Can you work these out from the model? Positions are in its coordinate system, mm. A direction names the side the tool comes from. Coordinates: 2 decimals unless noted, no trailing zeros. Order: outer loops, then holes, each group sorted by start corner. A loop starts at its lowest first (then second) coordinate and runs counter-clockwise, first axis right, second up. Notation, with made-up numbers: (51, -27.75) -> (109, -27.75) arc R27 ccw to (109, -9.75) -> close; hole circle Ø10 at (-32, 13.5). An arc over 180 degrees is marked (long way). Use a Markdown table: item, result. Add a question column.
1. For faces 1 (the conical face through (-34.713, -10.932, 38.782)), 2 (the flat face through (0, 0, 1.5)), 3 (the conical face through (-20.062, 38.572, 136.423)), which set-ups out of +Z, -Z, +X, -X, +Y, -Y let a thin tool reach every point of the face, with its end or its side?
2. Suppose I cut it at A-A, the plane z = 139. List the corners of the cut face in (x, y) for me.
3. We'd pull the mould along X, two halves only. Please class faces 4 (the conical face through (-38.15, 15.82, 81.86)), 5 (the flat face through (-21, -33, 160)), 6 (the conical face through (-38.22, -12.04, 82.72)): pulls with the +X half, pulls with the -X half, needs draft (parallel to the pull), parting line crosses it, or undercut.
4. For pin 1 Ø19 at (x, y) = (-11, -14.5) entering from +Z; pin 2 Ø12 at (y, z) = (-14.5, 39.5) entering from +X; pin 3 Ø1 at (y, z) = (9.5, 140) entering from +X, each with a flat end and sliding along its axis, tell me the tip position at first contact or that it passes through.
5. If I drill on line 1 along Z through (x, y) = (23, 8); line 2 along Y through (x, z) = (-31.5, 91); line 3 along X through (y, z) = (31.5, 58.5), over which ranges is the centre line in solid material (lowest first)? Write a range as from..to.
6. Suppose I cut it at B-B, the plane z = 31. List the corners of the cut face in (x, y) for me, then the cut area to 3 significant figures.
```python
from build123d import *

# Parameters (mm, degrees)
F2_R = 5
F3_T = -1.5


with BuildPart() as f1:
    # F0 (on Front) → F1 (revolve)
    with BuildSketch(Plane.XZ):
        Polygon((-40, 80), (-33.0009069179, 0), (0, 0), (0, 160), (-40, 160), (-53.0446591225, 98.6297039244), align=None)
    revolve(axis=Axis((0, 0, 80), (0, 0, 1)))

    # F2
    f2_edges = [f1.edges().sort_by_distance(p)[0] for p in [
        (53.044659, 0, 98.629704),
        (40, 0, 80),
    ]]
    fillet(f2_edges, radius=F2_R)

    # F3
    f3_openings = [f1.faces().sort_by_distance(p)[0] for p in [
        (0, 0, 160),
    ]]
    offset(amount=F3_T, openings=f3_openings)


solid = f1.part
```
Worked out:
| question | item | result |
|---|---|---|
| 1 | face 1 | -Z |
| 1 | face 2 | +Z |
| 1 | face 3 | none |
| 2 | outline | circle Ø88.93 at (0, 0); hole circle Ø85.86 at (0, 0) |
| 3 | face 4 | parting line crosses it |
| 3 | face 5 | needs draft |
| 3 | face 6 | undercut |
| 4 | pin 1 | stops at z = 1.5 |
| 4 | pin 2 | stops at x = 35.55 |
| 4 | pin 3 | stops at x = 43.37 |
| 5 | line 1 | z = 0..1.5 |
| 5 | line 2 | y = -35.82..-33.35, 33.35..35.82 |
| 5 | line 3 | x = -21.47..-18.66, 18.66..21.47 |
| 6 | outline | circle Ø71.43 at (0, 0); hole circle Ø68.41 at (0, 0) |
| 6 | area | 331 mm² |
